Source: three-view drawing plus pictorial views. Frame: mm from the lowest corner of the part. A direction names the side the tool comes from. Give positions to 0.01 mm unless a question says otherwise; leave off trailing zeros. Order: outer loops, then holes, each group sorted by start corner. A loop starts at its lowest first (then second) coordinate and runs counter-clockwise, first axis right, second up.
1) First-contact query: P1, Ø6, axis at x = 13, z = 6, coming from the +Y side; P2, Ø1, axis at y = 7, z = 19.5, coming from the -X side; P3, Ø12, axis at y = 16, z = 9.5, coming from the -X side; P4, Ø7.5, axis at x = 7.5, y = 7.5, coming from the +Z side. Flat tips, straight axial feed; report the tip coordinate or a pass-through.
2) Access query for the marked faces 1, 2 and 3. Directions: +Z, -Z, +X, -X, +Y, -Y. A direction counts if a zero-diameter tool reaches every point of the face in a straight line with its end or side. Return the directions, or none.
3) Section B-B, the plane z = 22.5. Return loops of the section in (x, y).
4) Draft query along Y for the marked faces 4, 5 and 6. Return one class per face: released by +Y, released by -Y, zero draft, split by the parting line, or undercut.
5) Section D-D, the plane y = 15.5. Return loops of the section in (x, z).
6) Section A-A, the plane x = 12.5. Return loops of the section in (y, z).
7) Material intervals for line 1 (Z direction, x = 21.25, y = 18); line 2 (Y direction, x = 12.5, z = 14); line 3 (Z direction, x = 15.1, y = 12.5), sorted ascending.
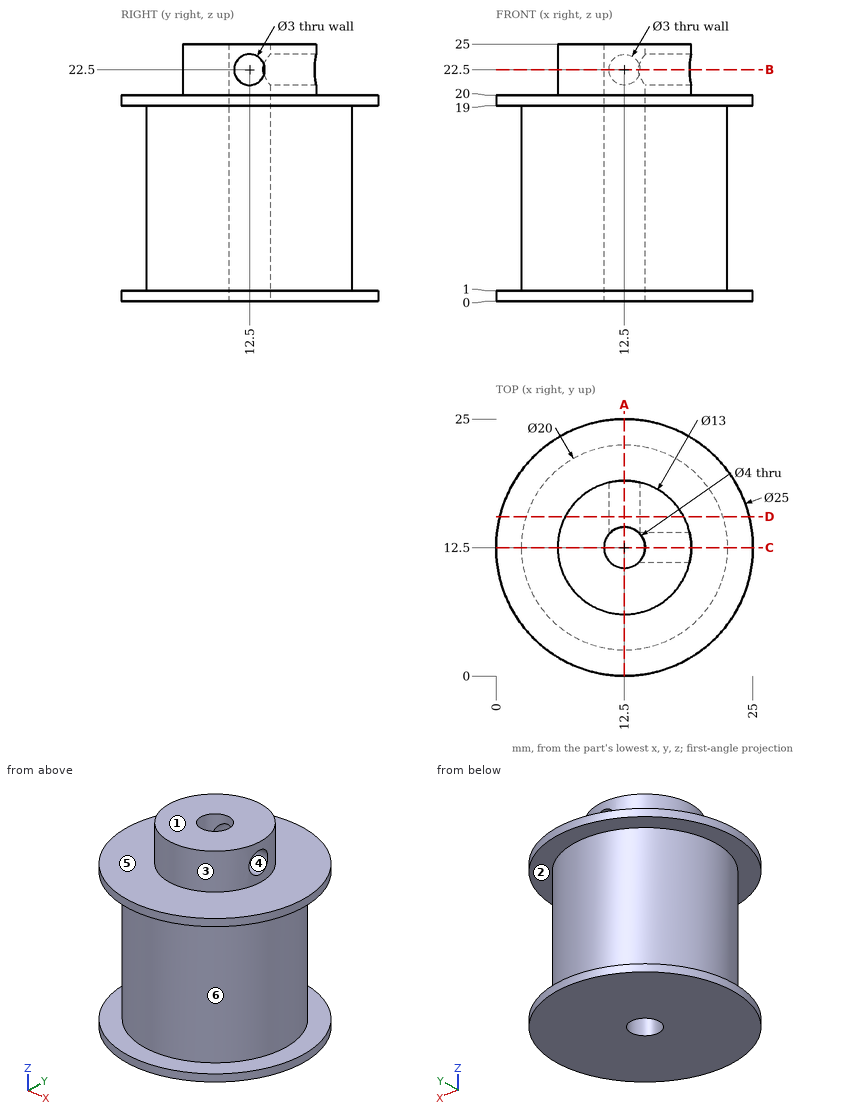
From the geometry:
1. P1: stops at y = 22.5
1. P2: stops at x = 1.04
1. P3: stops at x = 2.5
1. P4: stops at z = 25
2. face 1: +Z, +X, -X, +Y, -Y
2. face 2: none
2. face 3: +Z
3. outline: (11, 13.82) - (11, 18.82) arc R6.5 ccw (long way) to (18.82, 11) - (13.82, 11) arc R2 cw to start; (14, 14) - (18.82, 14) arc R6.5 ccw to (14, 18.82) - close
4. face 4: undercut
4. face 5: zero draft
4. face 6: split by the parting line
5. outline: (0.37, 0) - (24.63, 0) - (24.63, 1) - (22.04, 1) - (22.04, 19) - (24.63, 19) - (24.63, 20) - (18.27, 20) - (18.27, 25) - (6.73, 25) - (6.73, 20) - (0.37, 20) - (0.37, 19) - (2.96, 19) - (2.96, 1) - (0.37, 1) - close; hole circle Ø3 at (12.5, 22.5)
6. outline: (0, 0) - (10.5, 0) - (10.5, 25) - (6, 25) - (6, 20) - (0, 20) - (0, 19) - (2.5, 19) - (2.5, 1) - (0, 1) - close; (14.5, 0) - (25, 0) - (25, 1) - (22.5, 1) - (22.5, 19) - (25, 19) - (25, 20) - (19, 20) - (19, 21) - (14.5, 21) - close; (14.5, 24) - (19, 24) - (19, 25) - (14.5, 25) - close
7. line 1: z = 0 to 1, 19 to 20
7. line 2: y = 2.5 to 10.5, 14.5 to 22.5
7. line 3: z = 0 to 21, 24 to 25
